Source: CAD feature listing. Evaluate the final solid. Frame: model axes, mm. Round coordinates to 2 decimals unless told otherwise and drop trailing zeros. Write each loop counter-clockwise with the first axis right and the second up, starting at its lowest first coordinate (ties: lowest second). Pieces come first, ordered by that corner, then holes.
from build123d import *

# Parameters (mm, degrees)
SKETCH_3_W          = 98
SKETCH_3_H          = 150
EXTRUDE_1_DEPTH     = 3
FILLET_1_R          = 4
SKETCH_5_R          = 1.6
CUT_EXTRUDE_1_DEPTH = 3
SKETCH_6_R          = 1.6
CUT_EXTRUDE_2_DEPTH = 3
SKETCH_7_R          = 1.6
CUT_EXTRUDE_3_DEPTH = 3
SKETCH_8_R          = 1.6
CUT_EXTRUDE_4_DEPTH = 3
SKETCH_9_R          = 1.6
CUT_EXTRUDE_5_DEPTH = 10
SKETCH_10_R         = 1.6
CUT_EXTRUDE_6_DEPTH = 10
SKETCH_11_W         = 15
SKETCH_11_H         = 15
CUT_EXTRUDE_7_DEPTH = 10
FILLET_2_R          = 4


with BuildPart() as part:
    # 草图3 → 凸台-拉伸1 (new body)
    with BuildSketch(Plane(origin=(0, 0, 0), x_dir=(1, 0, 0), z_dir=(0, 1, 0))):
        Rectangle(SKETCH_3_W, SKETCH_3_H)
    extrude(amount=EXTRUDE_1_DEPTH)

    # 圆角1
    fillet_1_edges = [part.edges().sort_by_distance(p)[0] for p in [
        (49, 1.5, 75),
        (-49, 1.5, 75),
        (-49, 1.5, -75),
        (49, 1.5, -75),
    ]]
    fillet(fillet_1_edges, radius=FILLET_1_R)

    # 草图5 → 切除-拉伸1 (cut)
    with BuildSketch(Plane.XZ):
        with Locations(Location((-39, -47, 0), (0, 0, 270))):
            Circle(SKETCH_5_R)
        with Locations(Location((-25, -47, 0), (0, 0, 90))):
            Circle(SKETCH_5_R)
        with Locations(Location((-39, -63, 0), (0, 0, 90))):
            Circle(SKETCH_5_R)
        with Locations(Location((-25, -63, 0), (0, 0, 270))):
            Circle(SKETCH_5_R)
        with Locations(Location((25, -47, 0), (0, 0, 270))):
            Circle(SKETCH_5_R)
        with Locations(Location((25, -63, 0), (0, 0, 90))):
            Circle(SKETCH_5_R)
        with Locations(Location((39, -63, 0), (0, 0, 270))):
            Circle(SKETCH_5_R)
        with Locations(Location((39, -47, 0), (0, 0, 90))):
            Circle(SKETCH_5_R)
    extrude(amount=-CUT_EXTRUDE_1_DEPTH, mode=Mode.SUBTRACT)

    # 草图6 → 切除-拉伸2 (cut)
    with BuildSketch(Plane.XZ):
        with Locations(Location((-25, 60.5, 0), (0, 0, 270))):
            Circle(SKETCH_6_R)
        with Locations(Location((-25, 25.5, 0), (0, 0, 90))):
            Circle(SKETCH_6_R)
        with Locations(Location((25, 60.5, 0), (0, 0, 90))):
            Circle(SKETCH_6_R)
        with Locations(Location((25, 25.5, 0), (0, 0, 270))):
            Circle(SKETCH_6_R)
    extrude(amount=-CUT_EXTRUDE_2_DEPTH, mode=Mode.SUBTRACT)

    # 草图7 → 切除-拉伸3 (cut)
    with BuildSketch(Plane.XZ):
        with Locations(Location((-18.2, 8.2, 0), (0, 0, 270))):
            Circle(SKETCH_7_R)
        with Locations(Location((18.2, 8.2, 0), (0, 0, 90))):
            Circle(SKETCH_7_R)
        with Locations(Location((18.2, -28.2, 0), (0, 0, 270))):
            Circle(SKETCH_7_R)
        with Locations(Location((-18.2, -28.2, 0), (0, 0, 90))):
            Circle(SKETCH_7_R)
    extrude(amount=-CUT_EXTRUDE_3_DEPTH, mode=Mode.SUBTRACT)

    # 草图8 → 切除-拉伸4 (cut)
    with BuildSketch(Plane.XZ):
        with Locations(Location((45, 50, 0), (0, 0, 270))):
            Circle(SKETCH_8_R)
        with Locations(Location((-45, 50, 0), (0, 0, 90))):
            Circle(SKETCH_8_R)
        with Locations(Location((45, -20, 0), (0, 0, 90))):
            Circle(SKETCH_8_R)
        with Locations(Location((-45, -20, 0), (0, 0, 270))):
            Circle(SKETCH_8_R)
    extrude(amount=-CUT_EXTRUDE_4_DEPTH, mode=Mode.SUBTRACT)

    # 草图9 → 切除-拉伸5 (cut)
    with BuildSketch(Plane.XZ):
        with Locations(Location((-45, 35, 0), (0, 0, 270))):
            Circle(SKETCH_9_R)
        with Locations(Location((-45, 20, 0), (0, 0, 270))):
            Circle(SKETCH_9_R)
        with Locations(Location((45, 20, 0), (0, 0, 270))):
            Circle(SKETCH_9_R)
        with Locations(Location((45, 35, 0), (0, 0, 270))):
            Circle(SKETCH_9_R)
        with Locations(Location((-45, 10, 0), (0, 0, 270))):
            Circle(SKETCH_9_R)
        with Locations(Location((-45, -5, 0), (0, 0, 270))):
            Circle(SKETCH_9_R)
        with Locations(Location((45, 10, 0), (0, 0, 270))):
            Circle(SKETCH_9_R)
        with Locations(Location((45, -5, 0), (0, 0, 270))):
            Circle(SKETCH_9_R)
        with Locations(Location((-7.5, 71, 0), (0, 0, 270))):
            Circle(SKETCH_9_R)
        with Locations(Location((7.5, 71, 0), (0, 0, 270))):
            Circle(SKETCH_9_R)
        with Locations(Location((7.5, -71, 0), (0, 0, 270))):
            Circle(SKETCH_9_R)
        with Locations(Location((-7.5, -71, 0), (0, 0, 270))):
            Circle(SKETCH_9_R)
    extrude(amount=-CUT_EXTRUDE_5_DEPTH, mode=Mode.SUBTRACT)

    # 草图10 → 切除-拉伸6 (cut)
    with BuildSketch(Plane(origin=(0, 3, 0), x_dir=(1, 0, 0), z_dir=(0, 1, 0))):
        with Locations(Location((-15, 70.394924421, 0), (0, 0, 270))):
            Circle(SKETCH_10_R)
        with Locations(Location((15, 70.394924421, 0), (0, 0, 90))):
            Circle(SKETCH_10_R)
        with Locations(Location((-15, 40.394924421, 0), (0, 0, 90))):
            Circle(SKETCH_10_R)
        with Locations(Location((15, 40.394924421, 0), (0, 0, 270))):
            Circle(SKETCH_10_R)
    extrude(amount=-CUT_EXTRUDE_6_DEPTH, mode=Mode.SUBTRACT)

    # 草图11 → 切除-拉伸7 (cut)
    with BuildSketch(Plane(origin=(0, 3, 0), x_dir=(1, 0, 0), z_dir=(0, 1, 0))):
        with BuildLine():
            Line((-7.5, -59), (-7.5, 21))
            ThreePointArc((-7.5, 21), (0, 28.5), (7.5, 21))
            Line((7.5, 21), (7.5, -59))
            ThreePointArc((7.5, -59), (0, -66.5), (-7.5, -59))
        make_face()
        with Locations((0, 54.410429289)):
            Rectangle(SKETCH_11_W, SKETCH_11_H)
    extrude(amount=-CUT_EXTRUDE_7_DEPTH, mode=Mode.SUBTRACT)

    # 圆角2
    fillet_2_edges = [part.edges().sort_by_distance(p)[0] for p in [
        (7.5, 1.5, -61.910429289),
        (7.5, 1.5, -46.910429289),
        (-7.5, 1.5, -46.910429289),
        (-7.5, 1.5, -61.910429289),
    ]]
    fillet(fillet_2_edges, radius=FILLET_2_R)


solid = part.part
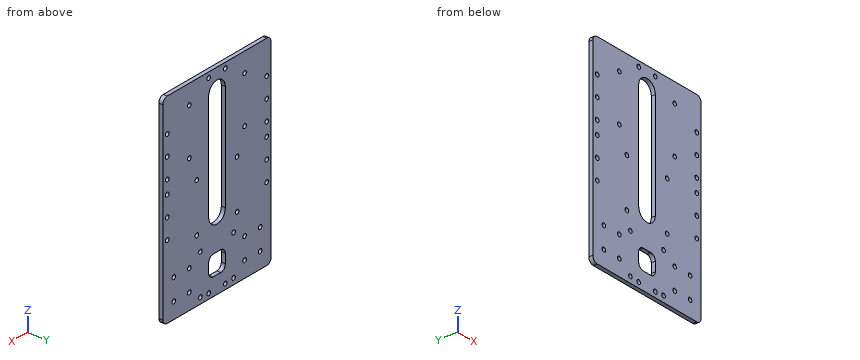
1) Section query D-D on y = 0.9. State how many separate pieces and enclosed holes the cut face has, then the cut area to 3 significant figures.
Taken from the geometry:
separate pieces: 1
enclosed holes: 38
area: 12,800 mm2
2) Contact query for a flat-ended pin moving along its axis: P1, Ø2, axis at x = -6, z = 37.5, coming from the +Y side. Output: stop coordinate, or through.
Taken from the geometry:
P1: passes through
3) Material intervals for line 1 (X direction, y = 2.2, z = 35); line 2 (X direction, y = 1.9, z = 25.5); line 3 (X direction, y = 2.1, z = -54), sorted ascending.
Taken from the geometry:
line 1: x = -49 to -46.6, -43.4 to -7.5, 7.5 to 43.4, 46.6 to 49
line 2: x = -49 to -26.6, -23.4 to -7.5, 7.5 to 23.4, 26.6 to 49
line 3: x = -49 to -7.5, 7.5 to 49
4) Section query C-C on z = 0.5. Return the cut outline in (x, y), then the cut area to 3 significant figures.
Taken from the geometry:
outline: (-49, 0) - (-7.5, 0) - (-7.5, 3) - (-49, 3) - close; (7.5, 0) - (49, 0) - (49, 3) - (7.5, 3) - close
area: 249 mm2
5) Section query B-B on x = -15. Return the cut outline in (y, z).
Taken from the geometry:
outline: (0, -75) - (3, -75) - (3, -71.99) - (0, -71.99) - close; (0, -68.79) - (3, -68.79) - (3, -41.99) - (0, -41.99) - close; (0, -38.79) - (3, -38.79) - (3, 75) - (0, 75) - close
6) Section query A-A on z = 35. Return the cut outline in (x, y).
Taken from the geometry:
outline: (-49, 0) - (-46.6, 0) - (-46.6, 3) - (-49, 3) - close; (-43.4, 0) - (-7.5, 0) - (-7.5, 3) - (-43.4, 3) - close; (7.5, 0) - (43.4, 0) - (43.4, 3) - (7.5, 3) - close; (46.6, 0) - (49, 0) - (49, 3) - (46.6, 3) - close
